```python
from build123d import *

# Parameters (mm, degrees)
SKETCH1_R                      = 32.5
BOSS_EXTRUDE1_DEPTH            = 5
CBORE_FOR_M4_SHCS1_D           = 4.5
CBORE_FOR_M4_SHCS1_CBORE_D     = 8.5
CBORE_FOR_M4_SHCS1_CBORE_DEPTH = 2.5
FILLET2_R                      = 1
FILLET3_R                      = 1


with BuildPart() as part:
    # Sketch1 → Boss-Extrude1 (new body)
    # profile 1 of 3: a face of its own
    with BuildSketch(Plane.XY):
        Circle(SKETCH1_R)
        with BuildLine():
            ThreePointArc((23, -5.63e-15), (17.621010186706098, -14.78174549909448), (3.9999999999999916, -22.64950330581225))
            Line((4, -22.64950330581225), (4.000000000000002, -29.732137494637012))
            ThreePointArc((4.0000000000000036, -29.73213749463701), (-3.6165626901756736, -29.781210088040908), (-11, -27.910571473905726))
            ThreePointArc((-11, -27.910571473905726), (-23.481565178581636, -18.6712639305437), (-29.671263930543617, -4.429006295324187))
            Line((-29.671263930543613, -4.429006295324186), (-22.9928556845359, -0.5732254967333699))
            ThreePointArc((-22.992855684535897, -0.5732254967333679), (-17.771682573326455, 14.600249946933266), (-3.899999999999999, 22.6669362729064))
            Line((-3.9, 22.6669362729064), (-3.9, 29.74541981549428))
            ThreePointArc((-3.8999999999999995, 29.74541981549428), (-1.204897673941924, 29.975793927689868), (1.4999999999999982, 29.96247653315726))
            ThreePointArc((1.4999999999999982, 29.96247653315726), (16.28027637225523, 25.19826583800932), (26.69826583800923, 13.682200160902106))
            Line((26.69826583800923, 13.682200160902106), (20.626179210300915, 10.176479311851942))
            ThreePointArc((20.626179210300908, 10.17647931185194), (22.398684356864813, 5.2248386655991155), (23, 0))
        make_face(mode=Mode.SUBTRACT)
    # profile 2 of 3: a face of its own
    with BuildSketch(Plane.XY):
        with BuildLine():
            ThreePointArc((1.4999999999999991, 22.951034835057), (12.774555523205114, 19.126179210300986), (20.626179210300908, 10.17647931185194))
            Line((20.626179210300915, 10.176479311851942), (26.69826583800923, 13.682200160902106))
            ThreePointArc((26.69826583800923, 13.682200160902106), (16.28027637225523, 25.19826583800932), (1.4999999999999982, 29.96247653315726))
            Line((1.5, 29.962476533157268), (1.5, 22.951034835057))
        make_face()
    # profile 3 of 3: a face of its own
    with BuildSketch(Plane.XY):
        with BuildLine():
            Line((-10.999999999999998, -27.910571473905723), (-11, -20.199009876724155))
            ThreePointArc((-11.000000000000004, -20.19900987672415), (-19.62578437999088, -11.992855684535943), (-22.992855684535897, -0.5732254967333679))
            Line((-22.9928556845359, -0.5732254967333699), (-29.671263930543613, -4.429006295324186))
            ThreePointArc((-29.671263930543617, -4.429006295324187), (-23.481565178581636, -18.6712639305437), (-11, -27.910571473905726))
        make_face()
    extrude(amount=-BOSS_EXTRUDE1_DEPTH)

    # CBORE for M4 SHCS1 (through all)
    with Locations(Plane(origin=(0, 0, -5), x_dir=(-1, 0, 0), z_dir=(0, 0, -1))):
        with Locations((27.328415146, 4.81873693), (9.491058977, 26.076470227), (-26.80444168, 7.182228502), (-9.491058977, -26.076470227)):
            CounterBoreHole(CBORE_FOR_M4_SHCS1_D / 2, CBORE_FOR_M4_SHCS1_CBORE_D / 2, CBORE_FOR_M4_SHCS1_CBORE_DEPTH)

    # Fillet2
    fillet2_edges = [part.edges().sort_by_distance(p)[0] for p in [
        (4.0000000000000036, -29.732137494637012, -2.5),
        (3.9999999999999947, -22.649503305812253, -2.5),
        (1.4999999999999996, 22.951034835057, -2.5),
        (1.4999999999999982, 29.96247653315727, -2.5),
        (-3.8999999999999995, 29.74541981549428, -2.5),
        (-3.9000000000000004, 22.666936272906405, -2.5),
        (-11.000000000000002, -20.199009876724155, -2.5),
        (-11, -27.910571473905723, -2.5),
    ]]
    fillet(fillet2_edges, radius=FILLET2_R)

    # Fillet3
    # the kernel refuses this fillet: 1 mm, written as the material it takes off along each edge
    with BuildSketch(Plane(origin=(0, 0, -5), x_dir=(1, 0, 0), z_dir=(0, -1, 0))) as fillet3_piece_1:
        with BuildLine():
            CenterArc((32.5 - FILLET3_R, FILLET3_R), FILLET3_R, 270, 90)
            Line((32.5 - FILLET3_R, 0), (32.5, 0))
            Line((32.5, 0), (32.5, FILLET3_R))
        make_face()
    revolve(axis=Axis((0, 0, -5), (0, 0, 1)), mode=Mode.SUBTRACT)
    with BuildSketch(Plane(origin=(-10.999999999999998, -27.22131517763241, -5), x_dir=(0, 0, 1), z_dir=(-2.3e-16, 1, 0))) as fillet3_piece_2:
        with BuildLine():
            CenterArc((FILLET3_R, -FILLET3_R), FILLET3_R, 90, 90)
            Line((0, -FILLET3_R), (0, 0))
            Line((0, 0), (FILLET3_R, 0))
        make_face()
    extrude(amount=6.436705486805881, mode=Mode.SUBTRACT)
    with BuildSketch(Plane(origin=(0, 8.9e-16, -5), x_dir=(-0.20416666666666677, 0.9789361430768722, 0), z_dir=(0.9789361430768722, 0.20416666666666677, 0))) as fillet3_piece_3:
        with BuildLine():
            CenterArc((23.000000000000007 + FILLET3_R, FILLET3_R), FILLET3_R, 180, 90.00000000000023)
            Line((23.000000000000007 + FILLET3_R, 0), (23.000000000000007, 0))
            Line((23.000000000000007, 0), (23.000000000000004, FILLET3_R))
        make_face()
    revolve(axis=Axis((0, 8.9e-16, -5), (0, 0, 1)), revolution_arc=138.21927913591307, mode=Mode.SUBTRACT)
    with BuildSketch(Plane(origin=(-3.354e-14, -2.2382e-13, -5), x_dir=(0.10344827586207093, -0.9946348346107555, 0), z_dir=(0.9946348346107555, 0.10344827586207093, 0))) as fillet3_piece_4:
        with BuildLine():
            CenterArc((29.999999999999787 + FILLET3_R, -FILLET3_R), FILLET3_R, 90, 90)
            Line((29.999999999999787 + FILLET3_R, 0), (29.999999999999787, 0))
            Line((29.999999999999787, 0), (29.999999999999787, -FILLET3_R))
        make_face()
    revolve(axis=Axis((-3.354e-14, -2.2382e-13, -5), (0, 0, -1)), revolution_arc=26.1090437980706, mode=Mode.SUBTRACT)
    with BuildSketch(Plane(origin=(4, -23.47338918861092, -5), x_dir=(0, 0, 1), z_dir=(2.5e-16, -1, 0))) as fillet3_piece_5:
        with BuildLine():
            CenterArc((FILLET3_R, -FILLET3_R), FILLET3_R, 90, 90)
            Line((0, -FILLET3_R), (0, 0))
            Line((0, 0), (FILLET3_R, 0))
        make_face()
    extrude(amount=5.371021015100997, mode=Mode.SUBTRACT)
    with BuildSketch(Plane(origin=(8.527e-14, 1.554e-14, -5), x_dir=(0.2083333333333306, -0.9780578828587924, 0), z_dir=(-0.9780578828587924, -0.2083333333333306, 0))) as fillet3_piece_6:
        with BuildLine():
            CenterArc((22.99999999999991 + FILLET3_R, FILLET3_R), FILLET3_R, 180, 89.99999999999977)
            Line((22.99999999999991 + FILLET3_R, 0), (22.99999999999991, 0))
            Line((22.99999999999991, 0), (22.999999999999915, FILLET3_R))
        make_face()
    revolve(axis=Axis((8.527e-14, 1.554e-14, -5), (0, 0, 1)), revolution_arc=161.9961440231332, mode=Mode.SUBTRACT)
    with BuildSketch(Plane(origin=(1.5, 28.995689334795948, -5), x_dir=(0, 0, 1), z_dir=(0, -1, 0))) as fillet3_piece_7:
        with BuildLine():
            CenterArc((FILLET3_R, -FILLET3_R), FILLET3_R, 90, 90)
            Line((0, -FILLET3_R), (0, 0))
            Line((0, 0), (FILLET3_R, 0))
        make_face()
    extrude(amount=5.126252810235989, mode=Mode.SUBTRACT)
    with BuildSketch(Plane(origin=(4.546e-14, -1.62004e-12, -5), x_dir=(-0.09999999999999602, 0.9949874371066204, 0), z_dir=(-0.9949874371066204, -0.09999999999999602, 0))) as fillet3_piece_8:
        with BuildLine():
            CenterArc((30.000000000001613 + FILLET3_R, -FILLET3_R), FILLET3_R, 90, 90)
            Line((30.000000000001613 + FILLET3_R, 0), (30.000000000001613, 0))
            Line((30.000000000001613, 0), (30.000000000001613, -FILLET3_R))
        make_face()
    revolve(axis=Axis((4.546e-14, -1.62004e-12, -5), (0, 0, -1)), revolution_arc=6.727077693922609, mode=Mode.SUBTRACT)
    with BuildSketch(Plane(origin=(-3.9, 23.494467433844935, -5), x_dir=(-4.4e-16, 0, 1), z_dir=(0, 1, 0))) as fillet3_piece_9:
        with BuildLine():
            CenterArc((FILLET3_R, -FILLET3_R), FILLET3_R, 90.00000000000003, 89.99999999999994)
            Line((4.4e-16, -FILLET3_R), (0, 0))
            Line((0, 0), (FILLET3_R, 0))
        make_face()
    extrude(amount=5.360168242247035, mode=Mode.SUBTRACT)
    with BuildSketch(Plane(origin=(-4.9, 23.49446743384493, -5), x_dir=(0.2041666666666649, -0.9789361430768725, 0), z_dir=(-0.9789361430768725, -0.2041666666666649, 0))) as fillet3_piece_10:
        with BuildLine():
            CenterArc((0.9999999999999997 - FILLET3_R, FILLET3_R), FILLET3_R, 270, 90)
            Line((0.9999999999999997 - FILLET3_R, 0), (0.9999999999999997, 0))
            Line((0.9999999999999997, 0), (0.9999999999999999, FILLET3_R))
        make_face()
    revolve(axis=Axis((-4.9, 23.49446743384493, -5), (0, 0, 1)), revolution_arc=78.2192791359134, mode=Mode.SUBTRACT)
    with BuildSketch(Plane(origin=(2.5, 23.86943652455996, -5), x_dir=(-0.10416666666666341, -0.9945598551900012, 0), z_dir=(0.9945598551900012, -0.10416666666666341, 0))) as fillet3_piece_11:
        with BuildLine():
            CenterArc((1 - FILLET3_R, -FILLET3_R), FILLET3_R, 0, 90)
            Line((1 - FILLET3_R, 0), (1, 0))
            Line((1, 0), (1, -FILLET3_R))
        make_face()
    revolve(axis=Axis((2.5, 23.86943652455996, -5), (0, 0, -1)), revolution_arc=84.02084320369887, mode=Mode.SUBTRACT)
    with BuildSketch(Plane(origin=(5.000000000000001, -23.47338918861092, -5), x_dir=(-1, 0, 0), z_dir=(0, -1, 0))) as fillet3_piece_12:
        with BuildLine():
            CenterArc((1 - FILLET3_R, -FILLET3_R), FILLET3_R, 0, 90)
            Line((1 - FILLET3_R, 0), (1, 0))
            Line((1, 0), (1, -FILLET3_R))
        make_face()
    revolve(axis=Axis((5.000000000000001, -23.47338918861092, -5), (0, 0, -1)), revolution_arc=77.97530081943442, mode=Mode.SUBTRACT)
    with BuildSketch(Plane(origin=(-12, -20.784609690826528, -5), x_dir=(1, 0, 0), z_dir=(0, -1, 0))) as fillet3_piece_13:
        with BuildLine():
            CenterArc((1 - FILLET3_R, FILLET3_R), FILLET3_R, 270, 90)
            Line((1 - FILLET3_R, 0), (1, 0))
            Line((1, 0), (1, FILLET3_R))
        make_face()
    revolve(axis=Axis((-12, -20.784609690826528, -5), (0, 0, 1)), revolution_arc=59.99999999999988, mode=Mode.SUBTRACT)
    with BuildSketch(Plane(origin=(-9.999999999999998, -27.221315177632405, -5), x_dir=(-0.34482758620689447, -0.9386660406080146, 0), z_dir=(0.9386660406080146, -0.34482758620689447, 0))) as fillet3_piece_14:
        with BuildLine():
            CenterArc((1.0000000000000018 + FILLET3_R, -FILLET3_R), FILLET3_R, 90, 90)
            Line((1.0000000000000018 + FILLET3_R, 0), (1.0000000000000018, 0))
            Line((1.0000000000000018, 0), (1.0000000000000018, -FILLET3_R))
        make_face()
    revolve(axis=Axis((-9.999999999999998, -27.221315177632405, -5), (0, 0, -1)), revolution_arc=69.82872865353495, mode=Mode.SUBTRACT)
    with BuildSketch(Plane(origin=(3.0000000000000013, -28.844410203711917, -5), x_dir=(1, 0, 0), z_dir=(0, 1, 0))) as fillet3_piece_15:
        with BuildLine():
            CenterArc((1.0000000000000004 + FILLET3_R, -FILLET3_R), FILLET3_R, 90, 90)
            Line((1.0000000000000004 + FILLET3_R, 0), (1.0000000000000004, 0))
            Line((1.0000000000000004, 0), (1.0000000000000004, -FILLET3_R))
        make_face()
    revolve(axis=Axis((3.0000000000000013, -28.844410203711917, -5), (0, 0, -1)), revolution_arc=84.06222754839449, mode=Mode.SUBTRACT)
    with BuildSketch(Plane(origin=(0.5, 28.995689334795948, -5), x_dir=(1, 0, 0), z_dir=(0, -1, 0))) as fillet3_piece_16:
        with BuildLine():
            CenterArc((1 + FILLET3_R, FILLET3_R), FILLET3_R, 180, 90)
            Line((1 + FILLET3_R, 0), (1, 0))
            Line((1, 0), (1, FILLET3_R))
        make_face()
    revolve(axis=Axis((0.5, 28.995689334795948, -5), (0, 0, 1)), revolution_arc=89.01209278334395, mode=Mode.SUBTRACT)
    with BuildSketch(Plane(origin=(-2.9, 28.85463567609197, -5), x_dir=(-0.09999999999999662, 0.9949874371066203, 0), z_dir=(0.9949874371066203, 0.09999999999999662, 0))) as fillet3_piece_17:
        with BuildLine():
            CenterArc((0.9999999999999991 + FILLET3_R, FILLET3_R), FILLET3_R, 180, 90)
            Line((0.9999999999999991 + FILLET3_R, 0), (0.9999999999999991, 0))
            Line((0.9999999999999991, 0), (0.9999999999999991, FILLET3_R))
        make_face()
    revolve(axis=Axis((-2.9, 28.85463567609197, -5), (0, 0, 1)), revolution_arc=84.26082952273342, mode=Mode.SUBTRACT)


solid = part.part
```
Input: part model. Units: mm. Frame: model coordinates. A direction names the side the tool comes from. Give positions to 0.01 mm unless a question says otherwise; leave off trailing zeros.
1) Contact query for flat-ended pins moving along their axis: pin 1 (2 mm diameter, centred on x = 25.5, z = -2, fed in from +Y); pin 2 (7 mm diameter, centred on x = -9.49, y = 26.08, fed in from -Z); pin 3 (2 mm diameter, centred on y = -24.5, z = -1.5, fed in from +X). Output: stop coordinate, or through.
A:
pin 1: stops at y = 21.35
pin 2: stops at z = -2.5
pin 3: stops at x = 22.45
2) Line query: L1, parallel to X at y = 28, z = -3.55; L2, parallel to X at y = -27.5, z = -0.65; L3, parallel to X at y = 7.5, z = -4.7. Output: solid intervals per line, ascending.
A:
L1: x = -16.5 to -13.28, -5.7 to -3.9, 1.5 to 16.5
L2: x = -17.32 to -10.96, 4 to 7.75, 11.23 to 17.32
L3: x = -31.33 to -30.63, -24.03 to -22.04, 22.04 to 22.57, 31.04 to 31.33
3) Mould query, pull axis X, two halves, no side actions, for faces 1 (the cylindrical face through (12.62, -23.2, -3.77)), 2 (the flat face through (15, 23, -5)). Classes: released by +X, released by -X, zero draft, split by the parting line, or undercut.
A:
face 1: undercut
face 2: zero draft
4) Reachability of faces 3 (the flat face through (2, 24, 0)), 4 (the flat face through (8, -28, -2.5)), 5 (the flat face through (-11, -24, -2)) from +Z, -Z, +X, -X, +Y, -Y: full face, straight path, thin tool, end or side. Return the list, or none.
A:
face 3: +Z, +X, -X, +Y, -Y
face 4: -Z
face 5: +Z, -Z
